Design review of the part built by this model. Coordinates are the model's own, in mm. A direction names the side the tool comes from. Give positions to 0.01 mm unless a question says otherwise; leave off trailing zeros. Write each loop counter-clockwise with the first axis right and the second up, starting at its lowest first coordinate (ties: lowest second). Pieces come first, ordered by that corner, then holes.
```python
from build123d import *

# Parameters (mm, degrees)
SKETCH_1_R          = 1.5
EXTRUDE_1_DEPTH     = 1
SKETCH_2_R          = 2
SKETCH_2_W          = 15
SKETCH_2_H          = 20
CUT_EXTRUDE_1_DEPTH = 315.198981539
SKETCH_3_W          = 130
SKETCH_3_H          = 76
CUT_EXTRUDE_2_DEPTH = 315.198981539
CUT_EXTRUDE_3_REACH = 293.112
FILLET_1_R          = 3


with BuildPart() as part:
    # 草图1 → 凸台-拉伸1 (new body)
    with BuildSketch(Plane.XY):
        Polygon((0, 0), (0, 76), (25, 76), (25, 116), (267, 116), (267, 76), (292, 76), (292, 0), align=None)
        with Locations((3, 48)):
            Circle(SKETCH_1_R, mode=Mode.SUBTRACT)
        with Locations((3, 28)):
            Circle(SKETCH_1_R, mode=Mode.SUBTRACT)
        with Locations(Location((289, 28, 0), (0, 0, 180))):
            Circle(SKETCH_1_R, mode=Mode.SUBTRACT)
        with Locations(Location((289, 48, 0), (0, 0, 180))):
            Circle(SKETCH_1_R, mode=Mode.SUBTRACT)
    extrude(amount=EXTRUDE_1_DEPTH)

    # 草图2 → 切除-拉伸1 (cut, through all)
    with BuildSketch(Plane.XY.offset(1)):
        with Locations((65, 111)):
            Circle(SKETCH_2_R)
        with Locations(Location((227, 111, 0), (0, 0, 180))):
            Circle(SKETCH_2_R)
        with Locations((146, 111)):
            Circle(SKETCH_2_R)
        with Locations((193.5, 106)):
            Rectangle(SKETCH_2_W, SKETCH_2_H)
        with Locations((98.5, 106)):
            Rectangle(SKETCH_2_W, SKETCH_2_H)
    extrude(amount=-CUT_EXTRUDE_1_DEPTH, mode=Mode.SUBTRACT)

    # 草图3 → 切除-拉伸2 (cut, through all)
    with BuildSketch(Plane.XY.offset(1)):
        with Locations((227, 38)):
            Rectangle(SKETCH_3_W, SKETCH_3_H)
    extrude(amount=-CUT_EXTRUDE_2_DEPTH, mode=Mode.SUBTRACT)

    # 草图4 → 切除-拉伸3 (cut, up to next)
    with BuildSketch(Plane.XY.offset(1), mode=Mode.PRIVATE) as cut_extrude_3_sk1:
        Polygon((30, 16), (75, 66), (30, 66), align=None)
    cut_extrude_3_tool1 = extrude(cut_extrude_3_sk1.sketch, amount=-CUT_EXTRUDE_3_REACH, mode=Mode.PRIVATE) & part.part
    # 草图4 → 切除-拉伸3 (cut, up to next)
    with BuildSketch(Plane.XY.offset(1), mode=Mode.PRIVATE) as cut_extrude_3_sk2:
        Polygon((86.180436071, 17.111111111), (86.180436071, 56), (51.180436071, 17.111111111), align=None)
    cut_extrude_3_tool2 = extrude(cut_extrude_3_sk2.sketch, amount=-CUT_EXTRUDE_3_REACH, mode=Mode.PRIVATE) & part.part
    # 草图4 → 切除-拉伸3 (cut, up to next)
    with BuildSketch(Plane.XY.offset(1), mode=Mode.PRIVATE) as cut_extrude_3_sk3:
        Polygon((121.180436071, 17.111111111), (86.180436071, 56), (86.180436071, 17.111111111), align=None)
    cut_extrude_3_tool3 = extrude(cut_extrude_3_sk3.sketch, amount=-CUT_EXTRUDE_3_REACH, mode=Mode.PRIVATE) & part.part
    # 草图4 → 切除-拉伸3 (cut, up to next)
    with BuildSketch(Plane.XY.offset(1), mode=Mode.PRIVATE) as cut_extrude_3_sk4:
        Polygon((97.360872141, 66), (142.360872141, 66), (142.360872141, 16), align=None)
    cut_extrude_3_tool4 = extrude(cut_extrude_3_sk4.sketch, amount=-CUT_EXTRUDE_3_REACH, mode=Mode.PRIVATE) & part.part
    add(cut_extrude_3_tool1.solids().sort_by_distance((45, 49.333333, 1))[0], mode=Mode.SUBTRACT)
    add(cut_extrude_3_tool2.solids().sort_by_distance((74.513769, 30.074074, 1))[0], mode=Mode.SUBTRACT)
    add(cut_extrude_3_tool3.solids().sort_by_distance((97.847103, 30.074074, 1))[0], mode=Mode.SUBTRACT)
    add(cut_extrude_3_tool4.solids().sort_by_distance((127.360872, 49.333333, 1))[0], mode=Mode.SUBTRACT)

    # 圆角1
    fillet_1_edges = [part.edges().sort_by_distance(p)[0] for p in [
        (121.180436071, 17.111111111, 0.5),
        (51.180436071, 17.111111111, 0.5),
        (86.180436071, 56, 0.5),
        (97.360872141, 66, 0.5),
        (142.360872141, 66, 0.5),
        (142.360872141, 16, 0.5),
        (75, 66, 0.5),
        (30, 16, 0.5),
        (30, 66, 0.5),
    ]]
    fillet(fillet_1_edges, radius=FILLET_1_R)


solid = part.part
```
(1) Clearance check with flat-ended pins moving along their axes: P1, Ø0.5, axis at x = 9, z = 0.5, coming from the +Y side; P2, Ø0.5, axis at y = 108.5, z = 0.5, coming from the -X side. State where each tip first meets the part, or that it passes through.
Resolved:
P1: stops at y = 76
P2: stops at x = 25
(2) Mouldability with a two-part tool opening along Y and no side actions: class faces 1 (the face through (52.615, 41.128, 0.507)), 2 (the face through (106, 72, 0)) as pulls with the +Y half, pulls with the -Y half, needs draft (parallel to the pull), parting line crosses it, or undercut.
Resolved:
face 1: undercut
face 2: needs draft
(3) Consider section A-A, the plane y = 103.5. Give the boundary of the cut face in (x, z).
Resolved:
outline: (25, 0) - (91, 0) - (91, 1) - (25, 1) - close; (106, 0) - (186, 0) - (186, 1) - (106, 1) - close; (201, 0) - (267, 0) - (267, 1) - (201, 1) - close
(4) To check wall thickness, follow L1, parallel to Y at x = 3, z = 0.2; L2, parallel to Y at x = 227, z = 0.65; L3, parallel to X at y = 36.5, z = 0.65. State the ranges of each line that lie inside material, in increasing order.
Resolved:
L1: y = 0 to 26.5, 29.5 to 46.5, 49.5 to 76
L2: y = 76 to 109, 113 to 116
L3: x = 0 to 30, 48.45 to 68.63, 103.73 to 123.91, 142.36 to 162
(5) Consider section B-B, the plane z = 0.75. Give the number of separate pieces and of enclosed holes in the cut face, then the cut area to 3 significant figures.
Resolved:
separate pieces: 1
enclosed holes: 8
area: 17,800 mm2
(6) Consider section C-C, the plane x = 249. Give the boundary of the cut face in (y, z).
Resolved:
outline: (76, 0) - (116, 0) - (116, 1) - (76, 1) - close
(7) Tool access review of faces 3 (the face through (106, 72, 1)), 4 (the face through (70.016, 38.04, 0.507)): name each direction out of +Z, -Z, +X, -X, +Y, -Y from which nothing blocks a thin tool from reaching the whole face with its end or side.
Resolved:
face 3: +Z, +X, -X, +Y, -Y
face 4: +Z, -Z
